Check sheet for the drawn part. Datum: minimum x, y, z corner. Units: mm. Give positions to 0.01 mm unless a question says otherwise; leave off trailing zeros. Loops run counter-clockwise (first coordinate to the right, second up) from the corner with the lowest first, then second, coordinate; pieces in that order, holes last.
1. Cross-section at B-B, the plane x = 38. Record the cut outline in (y, z).
2. Material ranges on L1, parallel to X at y = 11.6, z = 89.79 (3 decimals); L2, parallel to Z at x = 133.5, y = 11; L3, parallel to Y at x = 137, z = 61, recorded low to high.
3. Go/stop test with flat-tipped pins: pin 1 Ø4 at (y, z) = (7.5, 88.5) entering from +X; pin 2 Ø1 at (y, z) = (8, 26) entering from -X; pin 3 Ø3 at (x, y) = (180.5, 7) entering from +Z; pin 4 Ø3.5 at (x, z) = (133.535, 10.21) entering from -Y. Record where each tip stops, or that it passes through.
4. Cross-section at C-C, the plane z = 17. Record the cut outline in (x, y).
5. Cross-section at D-D, the plane x = 115. Record the cut outline in (y, z).
6. Cross-section at A-A, the plane y = 7.25. Record the cut outline in (x, z), plus the area to 3 significant figures.
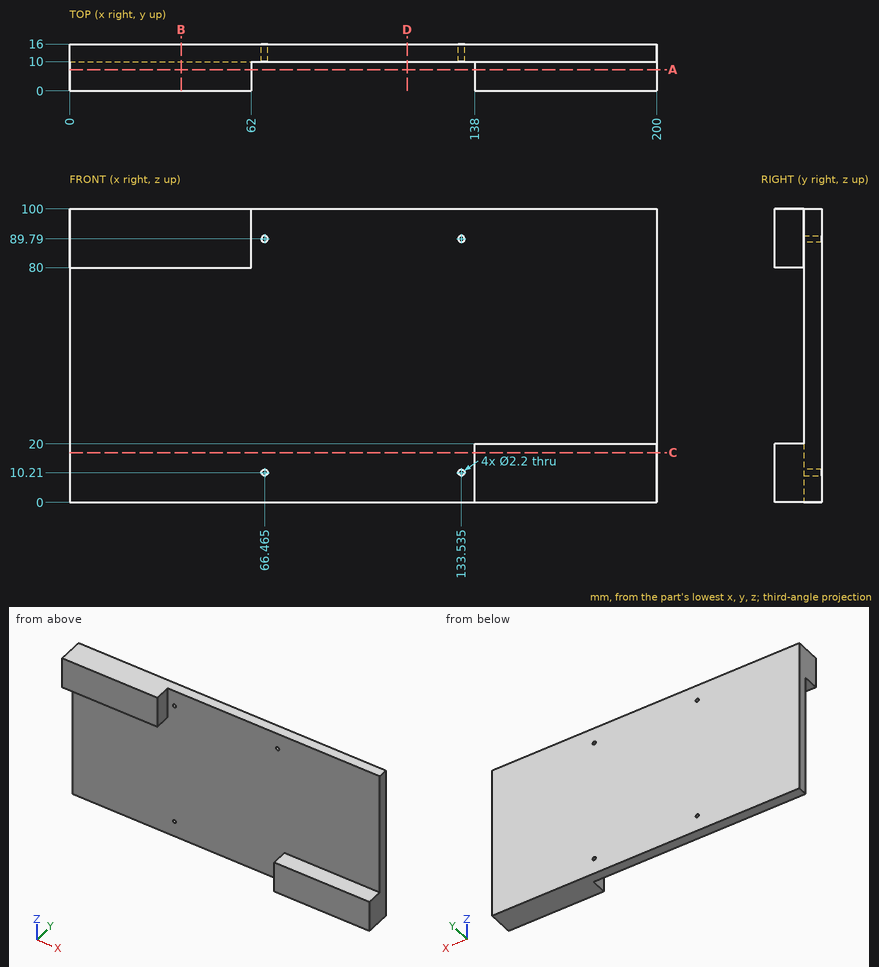
Result:
1. outline: (0, 80) - (10, 80) - (10, 0) - (16, 0) - (16, 100) - (0, 100) - close
2. L1: x = 0 to 65.365, 67.565 to 132.435, 134.635 to 200
2. L2: z = 0 to 9.11, 11.31 to 88.69, 90.89 to 100
2. L3: y = 10 to 16
3. pin 1: stops at x = 62
3. pin 2: passes through
3. pin 3: stops at z = 20
3. pin 4: stops at y = 10
4. outline: (0, 10) - (138, 10) - (138, 0) - (200, 0) - (200, 16) - (0, 16) - close
5. outline: (10, 0) - (16, 0) - (16, 100) - (10, 100) - close
6. outline: (0, 80) - (62, 80) - (62, 100) - (0, 100) - close; (138, 0) - (200, 0) - (200, 20) - (138, 20) - close
6. area: 2,480 mm2
